For this review, use the dimensioned drawing (mm, ordinates from the lowest corner) and the shaded views. A direction names the side the tool comes from. Give positions to 0.01 mm unless a question says otherwise; leave off trailing zeros. Order: outer loops, then holes, each group sorted by start corner. A loop starts at its lowest first (then second) coordinate and runs counter-clockwise, first axis right, second up. Notation, with made-up numbers: (11, 15) -> (66, 15) arc R26 cw to (66, 45) -> close; hole circle Ø10 at (60.25, -6). An arc over 180 degrees is marked (long way). One line per item, written item: value. Start each with the question number.
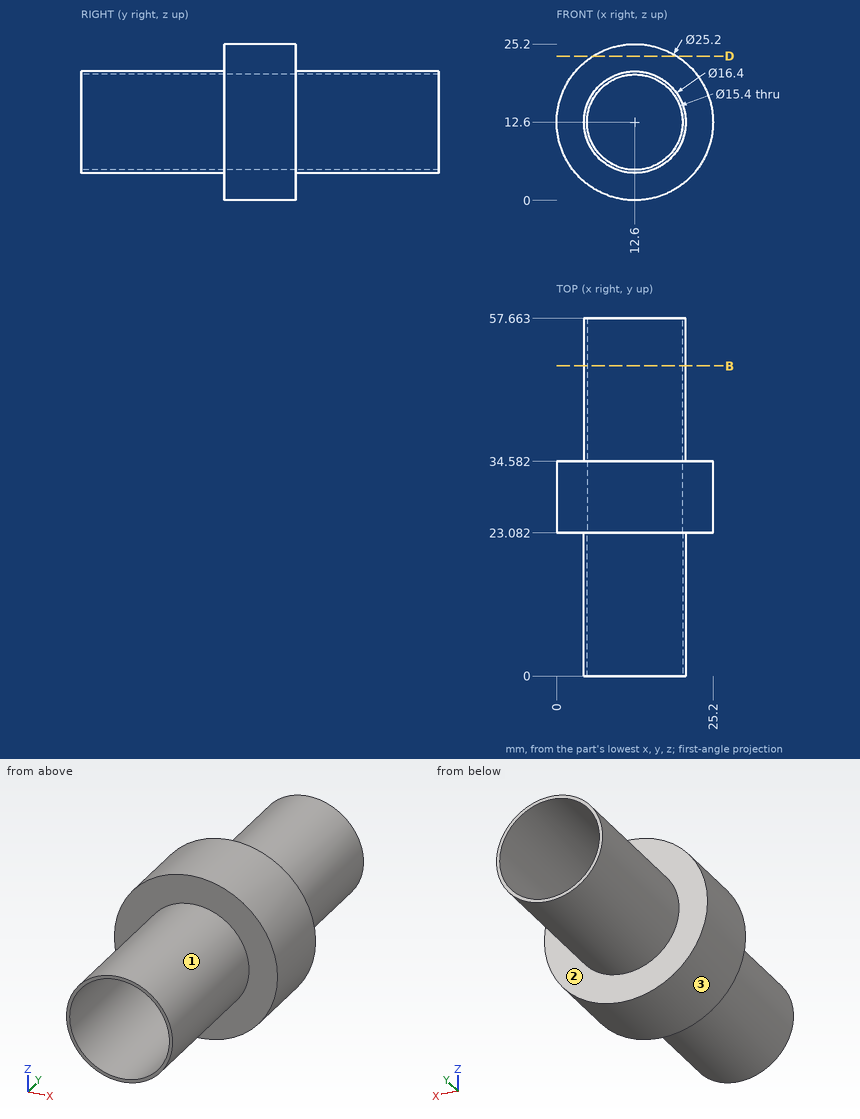
Q1. Take a section at D-D (z = 23.25). State the section outline as (x, y) points, and give its area (3 significant figures).
Q2. Take a section at B-B (y = 50). State the section outline as (x, z) points.
Q3. For pin 1 Ø7.5 at (x, z) = (16, 6.5) entering from -Y; pin 2 Ø8 at (y, z) = (50.5, 17.5) entering from -X; pin 3 Ø9 at (x, z) = (12.6, 12.6) entering from -Y; pin 4 Ø2 at (x, y) = (21, 15.5) entering from -Z (1 decimal), all flat-tipped, find the tip position at first contact; note any pin that passes through.
Q4. For the marked faces 1, 2 and 3, list the 3-axis set-ups (+Z, -Z, +X, -X, +Y, -Y) from which the entire face can be reached by the end or side of a thin tool; tool diameter is ignored.
Q5. For line 1 along X through (y, z) = (23.5, 12.6); line 2 along X through (y, z) = (48.5, 12.6), list the stretches that pass through material, from the lowest coordinate up.
Answers below:
1. outline: (5.87, 23.08) -> (19.33, 23.08) -> (19.33, 34.58) -> (5.87, 34.58) -> close
1. area: 155 mm²
2. outline: circle Ø16.4 at (12.6, 12.6); hole circle Ø15.4 at (12.6, 12.6)
3. pin 1: stops at y = 0
3. pin 2: stops at x = 4.45
3. pin 3: passes through
3. pin 4: stops at z = 9.1
4. face 1: -Y
4. face 2: +Y
4. face 3: +Y, -Y
5. line 1: x = 0 to 4.9, 20.3 to 25.2
5. line 2: x = 4.4 to 4.9, 20.3 to 20.8
